Geometry: final body of the model. Coordinates: model frame, mm. A direction names the side the tool comes from. Give positions to 0.01 mm unless a question says otherwise; leave off trailing zeros. Order: outer loops, then holes, each group sorted by start corner. A loop starts at its lowest first (then second) coordinate and runs counter-clockwise, first axis right, second up. Notation, with made-up numbers: (56, 27.25) - (75, 27.25) arc R6 cw to (75, 38.25) - close; hole circle Ø2 at (-36.75, 34.5). An arc over 180 degrees is marked (long way). Put each result on its own line as item: value. Start each with the question number.
1. Section B-B on x = 8.75. Return the cut outline in (y, z), plus the area to 3 significant figures.
2. Set-up query: faces 1 (the flat face through (15.93, 8.905, 25.165)), 2 (the flat face through (21, 28, 23)), 3 (the flat face through (16, 10, 7)), 4 (the flat face through (5.4, 6.8, 26.7)), 5 (the cylindrical face through (10.353, 27.226, 7.73)). Return all of +Z, -Z, +X, -X, +Y, -Y with unobstructed straight access to the full face (end or side cutting, diameter ignored); none if empty.
3. Section D-D on x = 13.5. Return the cut outline in (y, z), plus the area to 3 significant figures.
4. Section C-C on z = 15. Return the cut outline in (x, y), plus the area to 3 significant figures.
5. Mould query, pull axis Z, two halves, no side actions, for faces 6 (the flat face through (5, 20, 2.7)), 7 (the flat face through (16, 7, 14)), 8 (the cylindrical face through (15.93, 29.147, 5.763)), 9 (the flat face through (21, 28, 7)). Classes: pulls with the +Z half, pulls with the -Z half, needs draft (parallel to the pull), parting line crosses it, or undercut.
6. Ray query, line 1 along X through (y, z) = (3.1, 14); line 2 along Z through (x, y) = (1.75, 29); line 3 along X through (y, z) = (15.5, 2). Return the intervals inside material, ascending. Write a range as from..to.
7. Section A-A on y = 20. Return the cut outline in (x, z), plus the area to 3 significant figures.
8. First-contact query: P1, Ø10, axis at x = 5.5, z = 5, coming from the -Y side; P2, Ø2, axis at x = 10.5, z = 25, coming from the +Y side; P3, Ø5, axis at x = 15, y = 19, coming from the +Z side; P4, Ø9, axis at x = 17, y = 4.5, coming from the -Z side. Flat tips, straight axial feed; report the tip coordinate or a pass-through.
from build123d import *

# Parameters (mm, degrees)
CROQUIS1_R              = 10
SALIENTE_EXTRUIR1_DEPTH = 11
CROQUIS2_R              = 10
SALIENTE_EXTRUIR2_DEPTH = 10
CORTAR_EXTRUIR3_START   = -10
CORTAR_EXTRUIR3_DEPTH   = 10
CROQUIS8_R              = 1.55
CORTAR_EXTRUIR4_DEPTH   = 5
CORTAR_EXTRUIR8_REACH   = 52.656
CORTAR_EXTRUIR9_START   = -10
CORTAR_EXTRUIR9_DEPTH   = 10


with BuildPart() as part:
    # Croquis1 → Saliente-Extruir1 (new body)
    with BuildSketch(Plane(origin=(0, 0, 0), x_dir=(0, 0, -1), z_dir=(1, 0, 0))):
        with BuildLine():
            Line((-5.780776406, 0), (-24.219223594, 0))
            ThreePointArc((-24.219223594, 0), (-24.834635803, 0.211794562), (-25.189366094, 0.757464375))
            Line((-25.189366094, 0.757464375), (-28.235294118, 12.941176471))
            ThreePointArc((-28.235294118, 12.941176471), (-15, 35), (-1.764705882, 12.941176471))
            Line((-1.764705882, 12.941176471), (-4.810633906, 0.757464375))
            ThreePointArc((-4.810633906, 0.757464375), (-5.165364197, 0.211794562), (-5.780776406, 0))
        make_face()
        with Locations((-15, 20)):
            Circle(CROQUIS1_R, mode=Mode.SUBTRACT)
    extrude(amount=SALIENTE_EXTRUIR1_DEPTH)

    # Croquis2 → Saliente-Extruir2 (add)
    with BuildSketch(Plane(origin=(11, 0, 0), x_dir=(0, 0, -1), z_dir=(1, 0, 0))):
        with BuildLine():
            Line((-23.438447187, 2), (-6.561552813, 2))
            Line((-6.561552813, 2), (-3.643105675, 13.673788552))
            ThreePointArc((-3.643105675, 13.673788552), (-15, 33), (-26.356894325, 13.673788552))
            Line((-26.356894325, 13.673788552), (-23.438447187, 2))
        make_face()
        with Locations((-15, 20)):
            Circle(CROQUIS2_R, mode=Mode.SUBTRACT)
    extrude(amount=SALIENTE_EXTRUIR2_DEPTH)

    # Croquis3 → Cortar-Extruir3 (cut)
    with BuildSketch(Plane(origin=(21, 0, 0), x_dir=(0, 0, -1), z_dir=(1, 0, 0)).offset(CORTAR_EXTRUIR3_START)):
        Polygon((-9.561552813, 2), (-9.561552813, 10), (-4.561552813, 10), (-6.561552813, 2), align=None)
        with BuildLine():
            Line((-23.438447187, 2), (-18.438447187, 2))
            Line((-18.438447187, 2), (-18.438447187, 6.945227656))
            Line((-18.438447187, 6.945227656), (-18.438447187, 7.462971606))
            ThreePointArc((-18.438447187, 7.462971606), (-21.059353424, 8.498511571), (-23.395524099, 10.074518898))
            Line((-23.395524099, 10.074518898), (-23.194590952, 9.270786312))
            Line((-23.194590952, 9.270786312), (-21.876894374, 4))
            Line((-21.876894374, 4), (-23.938447187, 4))
            Line((-23.938447187, 4), (-23.438447187, 2))
        make_face()
    extrude(amount=CORTAR_EXTRUIR3_DEPTH, mode=Mode.SUBTRACT)

    # Croquis8 → Cortar-Extruir4 (cut)
    with BuildSketch(Plane.XZ.offset(-2)):
        with Locations(Location((16, 14, 0), (0, 0, 270))):
            Circle(CROQUIS8_R)
    extrude(amount=-CORTAR_EXTRUIR4_DEPTH, mode=Mode.SUBTRACT)

    # Croquis10 → Cortar-Extruir8 (cut, up to next)
    with BuildSketch(Plane.ZY, mode=Mode.PRIVATE) as cortar_extruir8_sk1:
        with BuildLine():
            Line((15, 32.3), (20.5, 32.3))
            Line((20.5, 32.3), (20.5, 28.649421946))
            ThreePointArc((20.5, 28.649421946), (22.247844507, 27.247844507), (23.649421946, 25.5))
            Line((23.649421946, 25.5), (27.3, 25.5))
            Line((27.3, 25.5), (27.3, 20))
            Line((27.3, 20), (27.3, 14.5))
            Line((27.3, 14.5), (23.649421946, 14.5))
            ThreePointArc((23.649421946, 14.5), (15, 9.75), (6.350578054, 14.5))
            Line((6.350578054, 14.5), (2.7, 14.5))
            Line((2.7, 14.5), (2.7, 20))
            Line((2.7, 20), (2.7, 25.5))
            Line((2.7, 25.5), (6.350578054, 25.5))
            ThreePointArc((6.350578054, 25.5), (7.752155493, 27.247844507), (9.5, 28.649421946))
            Line((9.5, 28.649421946), (9.5, 32.3))
            Line((9.5, 32.3), (15, 32.3))
        make_face()
    cortar_extruir8_tool1 = extrude(cortar_extruir8_sk1.sketch, amount=-CORTAR_EXTRUIR8_REACH, mode=Mode.PRIVATE) & part.part
    add(cortar_extruir8_tool1.solids().sort_by_distance((0, 20.746773, 15))[0], mode=Mode.SUBTRACT)

    # Croquis12 → Cortar-Extruir9 (cut)
    with BuildSketch(Plane(origin=(21, 0, 0), x_dir=(0, 0, -1), z_dir=(1, 0, 0)).offset(CORTAR_EXTRUIR9_START)):
        with BuildLine():
            Line((-19.208325083, 32.3), (-10.791674918, 32.3))
            ThreePointArc((-10.791674918, 32.3), (-15, 33), (-19.208325083, 32.3))
        make_face()
        with BuildLine():
            Line((-27.3, 15.791674917), (-27.3, 24.208325082))
            ThreePointArc((-27.3, 24.208325082), (-28, 20), (-27.3, 15.791674917))
        make_face()
        with BuildLine():
            Line((-2.7, 24.208325083), (-2.7, 15.791674917))
            ThreePointArc((-2.7, 15.791674917), (-2, 20), (-2.7, 24.208325083))
        make_face()
    extrude(amount=CORTAR_EXTRUIR9_DEPTH, mode=Mode.SUBTRACT)


solid = part.part
Resolved:
1. outline: (0, 5.78) arc R1 ccw to (0.76, 4.81) - (12.94, 1.76) arc R15 ccw (long way) to (12.94, 28.24) - (0.76, 25.19) arc R1 ccw to (0, 24.22) - close; hole (14.5, 2.7) - (25.5, 2.7) - (25.5, 6.35) arc R10.25 ccw to (28.65, 9.5) - (32.3, 9.5) - (32.3, 20.5) - (28.65, 20.5) arc R10.25 ccw to (25.5, 23.65) - (25.5, 27.3) - (14.5, 27.3) - (14.5, 23.65) arc R10.25 ccw to (14.5, 6.35) - close
1. area: 443 mm^2
2. face 1: +Z, +X, -Y
2. face 2: +Z, -Z, +X, +Y, -Y
2. face 3: -Z, +X, -Y
2. face 4: +Z, +X, -X, -Y
2. face 5: +X, -X
3. outline: (2, 9.56) - (10, 9.56) - (10, 4.56) - (13.67, 3.64) arc R13 ccw to (14.5, 3.22) - (14.5, 6.35) arc R10.25 cw to (14.5, 23.65) - (14.5, 26.78) arc R13 ccw to (13.67, 26.36) - (4, 23.94) - (4, 21.88) - (10.07, 23.4) arc R13 ccw to (7.46, 18.44) - (2, 18.44) - close; (25.5, 3.22) arc R13 ccw to (31.78, 9.5) - (28.65, 9.5) arc R10.25 cw to (25.5, 6.35) - close; (25.5, 23.65) arc R10.25 cw to (28.65, 20.5) - (31.78, 20.5) arc R13 ccw to (25.5, 26.78) - close
3. area: 169 mm^2
4. outline: (0, 0) - (11, 0) - (11, 2) - (14.82, 2) - (14.82, 7) - (17.18, 7) - (17.18, 2) - (21, 2) - (21, 9.75) - (0, 9.75) - close; (0, 32.3) - (11, 32.3) - (11, 35) - (0, 35) - close
4. area: 203 mm^2
5. face 6: undercut
5. face 7: undercut
5. face 8: pulls with the -Z half
5. face 9: needs draft
6. line 1: 0..14.45, 17.55..21
6. line 2: 3..9.5, 20.5..27
6. line 3: 0..11
7. outline: (0, 0) - (11, 0) - (11, 2.7) - (0, 2.7) - close; (0, 27.3) - (11, 27.3) - (11, 30) - (0, 30) - close
7. area: 59.4 mm^2
8. P1: y = 0
8. P2: y = 32
8. P3: through
8. P4: z = 9.56
